The drawing under review shows one solid part. Ordinate dimensions are in mm from its lowest x, y, z. Give positions to 0.01 mm unless a question says otherwise; leave off trailing zeros. Order: outer loops, then holes, each group sorted by start corner. A loop starts at its lowest first (then second) coordinate and runs counter-clockwise, first axis right, second up. Notation, with made-up numbers: (14.5, -3) - (40.5, -3) arc R27 cw to (40.5, 23) - close; hole circle Ø1 at (-28, -29). An arc over 180 degrees is marked (long way). Use CSV: the item, a comma, the result in double quotes. Start each with the question number.
1. To check wall thickness, follow line 1 (X direction, y = 8, z = 5) (1 decimal); line 2 (Y direction, x = 1.5, z = 40); line 3 (Z direction, x = 3.75, y = 8.5). State the ranges of each line that lie inside material, in increasing order. Write a range as [from, to].
2. Draft analysis for pull direction X (two halves, no side actions). For the marked faces 1, 2, 3 and 4, state which applies: released by +X, released by -X, zero draft, split by the parting line, or undercut.
3. Take a section at A-A, the plane z = 45. State the section outline as (x, y) points (1 decimal).
4. For pin 1 (1 mm diameter, centred on x = 5.5, z = 40, fed in from -Y); pin 2 (0.5 mm diameter, centred on x = 12, z = 27.5, fed in from -Y); pin 3 (2.5 mm diameter, centred on x = 5, y = 12, fed in from -Z), all flat-tipped, find the tip position at first contact; note any pin that passes through.
5. Take a section at B-B, the plane y = 1.75. State the section outline as (x, z) points (1 decimal).
6. Take a section at D-D, the plane y = 7.75. State the section outline as (x, z) points (1 decimal).
7. Take a section at C-C, the plane z = 26.5. State the section outline as (x, y) points (1 decimal), then the cut area to 3 significant figures.
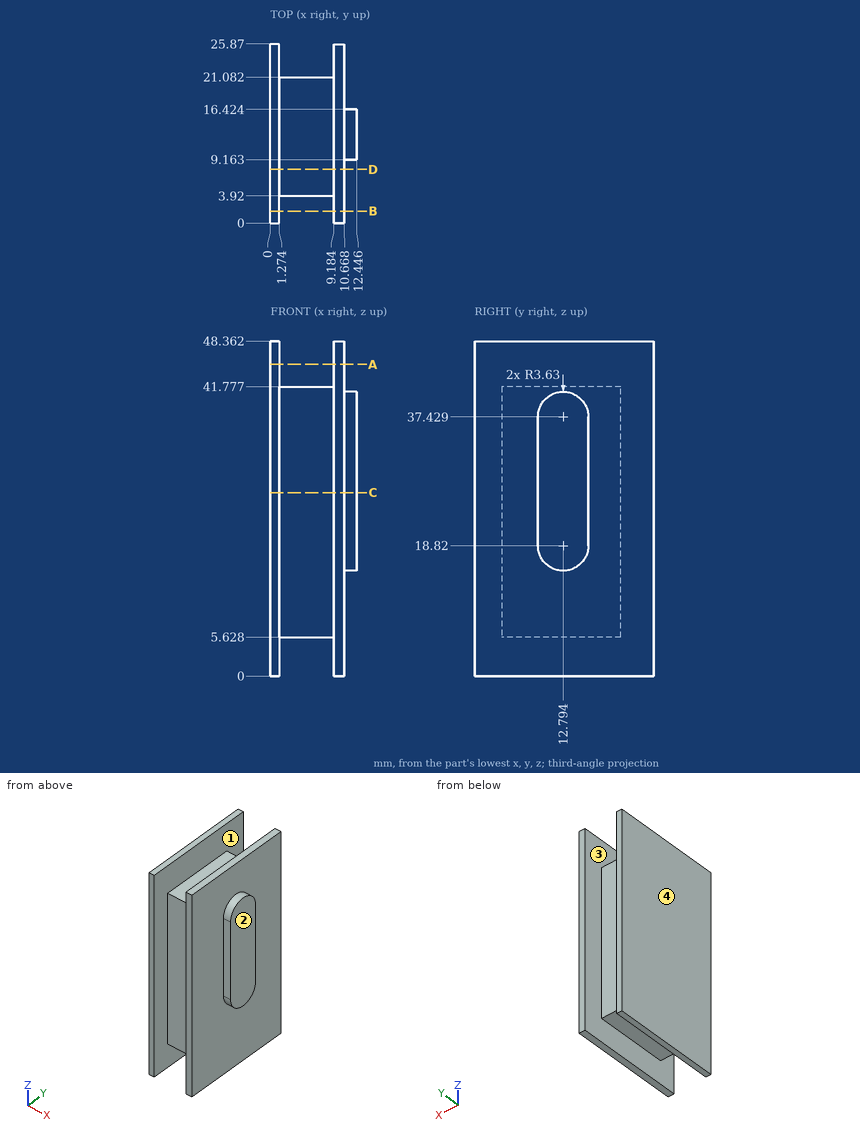
Determined:
1,line 1,"x = [0, 1.3], [9.2, 10.7]"
1,line 2,"y = [3.92, 21.08]"
1,line 3,"z = [5.63, 41.78]"
2,face 1,"undercut"
2,face 2,"released by +X"
2,face 3,"undercut"
2,face 4,"released by -X"
3,outline,"(0, 0) - (1.3, 0) - (1.3, 25.9) - (0, 25.9) - close; (9.2, 0) - (10.7, 0) - (10.7, 25.9) - (9.2, 25.9) - close"
4,pin 1,"stops at y = 3.92"
4,pin 2,"stops at y = 9.16"
4,pin 3,"stops at z = 5.63"
5,outline,"(0, 0) - (1.3, 0) - (1.3, 48.4) - (0, 48.4) - close; (9.2, 0) - (10.7, 0) - (10.7, 48.4) - (9.2, 48.4) - close"
6,outline,"(0, 0) - (1.3, 0) - (1.3, 5.6) - (9.2, 5.6) - (9.2, 0) - (10.7, 0) - (10.7, 48.4) - (9.2, 48.4) - (9.2, 41.8) - (1.3, 41.8) - (1.3, 48.4) - (0, 48.4) - close"
7,outline,"(0, 0) - (1.3, 0) - (1.3, 3.9) - (9.2, 3.9) - (9.2, 0) - (10.7, 0) - (10.7, 9.2) - (12.4, 9.2) - (12.4, 16.4) - (10.7, 16.4) - (10.7, 25.9) - (9.2, 25.9) - (9.2, 21.1) - (1.3, 21.1) - (1.3, 25.9) - (0, 25.9) - close"
7,area,"220 mm²"
